Autodesk Inventor part; units mm, degrees
ref_plane "YZ Plane" through (0, 0, 0) normal (1, 0, 0) x (0, 1, 0)
ref_plane "XZ Plane" through (0, 0, 0) normal (0, 1, 0) x (-1, 0, 0)
ref_plane "XY Plane" through (0, 0, 0) normal (0, 0, 1) x (1, 0, 0)
sketch "Szkic1" plane through (0, 0, 0) normal (0, 0, 1) x (1, 0, 0)
  circle A0 centre (0, 0) radius 40
  circle A1 centre (0, 0) radius 53
  dimension "d0" = 80
  dimension "d1" = 13
extrude "Wyciągnięcie proste1" add sketch "Szkic1" along normal blind 5
sketch "Szkic2" plane through (0, 0, 5) normal (0, 0, 1) x (1, 0, 0)
  circle A0 centre (0, 0) radius 40
  circle A1 centre (0, 0) radius 43
  dimension "d4" = 3
extrude "Wyciągnięcie proste2" add sketch "Szkic2" along normal blind 41.5
sketch "Szkic3" plane through (0, 0, 5) normal (0, 0, 1) x (1, 0, 0)
  circle A0 centre (0, 0) radius 43
  line L0 (0, 43) -> (0, 53)
  circle A1 centre (0, 0) radius 53
  line L1 (43, 0) -> (53, 0)
  line L2 (0, -43) -> (0, -53)
  line L3 (-43, 0) -> (-53, 0)
  point P0 (0, 48)
  point P1 (-48, 0)
  point P2 (0, -48)
  point P3 (48, 0)
hole "Otwór1" at (0, 48, 5) at (-48, 0, 5) at (0, -48, 5) at (48, 0, 5) direction (0, 0, -1) diameter 3.242 end through all countersink diameter 8 countersink angle 90
sketch "Szkic8" plane through (0, 0, 0) normal (0, 0, -1) x (-1, 0, 0)
  circle A0 centre (0, 0) radius 10.75
  line L0 (0, 0) -> (17, 0)
  line L1 (17, 0) -> (14.59, 0)
  line L2 (14.59, 0) -> (14.59, 5)
  line L3 (14.59, 0) -> (14.59, -5)
  circle A1 centre (14.59, 5) radius 1.621
  circle A2 centre (14.59, -5) radius 1.621
  line L4 (14.59, 5) -> (-35.19, 5)
  line L5 (14.59, -5) -> (-35.19, -5)
  circle A3 centre (-35.19, 5) radius 1.621
  circle A4 centre (-35.19, -5) radius 1.621
  line L6 (-33.569, -5) -> (-31.569, -5)
  line L7 (-31.569, -5) -> (-31.569, 5)
  line L8 (-35.19, 6.621) -> (-35.19, 8.621)
  line L9 (-35.19, 8.621) -> (-31.569, 8.621)
  line L10 (-31.569, 8.621) -> (-31.569, 5)
  line L11 (-36.811, 5) -> (-38.811, 5)
  line L12 (-35.19, -6.621) -> (-35.19, -8.621)
  line L13 (-35.19, -8.621) -> (-31.569, -8.621)
  line L14 (-31.569, -8.621) -> (-31.569, -5)
  line L15 (-35.19, -8.621) -> (-38.811, -8.621)
  line L16 (-38.811, 5) -> (-38.811, 8.621)
  line L17 (-38.811, 8.621) -> (-35.19, 8.621)
  line L18 (12.969, -5) -> (10.969, -5)
  line L19 (14.59, -6.621) -> (14.59, -8.621)
  line L20 (10.969, -5) -> (10.969, -8.621)
  line L21 (10.969, -8.621) -> (14.59, -8.621)
  line L22 (14.59, 6.621) -> (14.59, 8.621)
  line L23 (14.59, 8.621) -> (10.969, 8.621)
  line L24 (10.969, 8.621) -> (10.969, -5)
  line L25 (16.211, -5) -> (18.211, -5)
  line L26 (14.59, -8.621) -> (18.211, -8.621)
  line L27 (18.211, -8.621) -> (18.211, 8.621)
  line L28 (18.211, 8.621) -> (14.59, 8.621)
  circle A5 centre (0, 0) radius 40
  line L29 (-38.811, -8.621) -> (-39.0599, -8.621)
  line L30 (-38.811, 8.621) -> (-39.0599, 8.621)
  line L31 (-31.569, 8.621) -> (-30.569, 8.621)
  line L32 (-30.569, 8.621) -> (-30.569, -8.621)
  line L33 (-30.569, -8.621) -> (-31.569, -8.621)
  dimension "d59" = 3.242
  dimension "d54" = 21.5
  dimension "d55" = 17
  dimension "d56" = 2.41
  dimension "d57" = 5
  dimension "d58" = 5
  dimension "d60" = 3.242
  dimension "d61" = 49.78
  dimension "d62" = 3.242
  dimension "d63" = 3.242
  dimension "d64" = 2
  dimension "d66" = 2
  dimension "d67" = 2
  dimension "d68" = 2
  dimension "d69" = 2
  dimension "d70" = 2
  dimension "d71" = 2
  dimension "d74" = 49.78
  dimension "d87" = 1
extrude "Wyciągnięcie proste6" add sketch "Szkic8" against normal blind 32 contours L24 L4 A1 L2 L0 | L0 L3 A2 L5 L24 | L24 L23 L22 A1 L4 | L5 A2 L19 L21 L20 | L2 A1 L22 L28 L27 L25 A2 L3 | L7 L5 A4 L12 L15 L29 A5 L30 L16 L11 A3 L4 | L4 A3 L8 L9 L10 | L14 L13 L12 A4 L5 | A2 L25 L27 L26 L19 | A3 L11 L16 L17 L8
sketch "Szkic9" plane through (0, 0, 0) normal (0, 0, -1) x (-1, 0, 0)
  line L0 (11.0032, 0) -> (10.969, -1.9997)
  line L1 (10.969, -8.621) -> (10.969, 8.621)
  line L2 (10.969, -1.9997) -> (10.969, 2.0003)
  line L3 (10.969, 2.0003) -> (-31.569, 2.0003)
  line L4 (-31.569, -8.621) -> (-31.569, 8.621)
  line L5 (10.969, -1.9997) -> (-31.569, -1.9997)
  circle A0 centre (14.59, -5) radius 1.621
  line L6 (14.59, -5) -> (14.59, -8.621)
  line L7 (18.211, -8.621) -> (10.969, -8.621)
  line L8 (14.59, -8.621) -> (12.59, -8.621)
  line L9 (12.59, -8.621) -> (16.59, -8.621)
  line L10 (16.59, -8.621) -> (16.59, -36.3974)
  arc A1 (-39.0599, -8.621) -> (-39.0599, 8.621) centre (0, 0) ccw
  line L11 (12.59, -8.621) -> (12.59, -37.967)
  line L12 (10.969, 8.621) -> (18.211, 8.621)
  line L13 (12.59, 8.621) -> (12.59, 45.8086)
  line L14 (12.59, 8.621) -> (49.7776, 8.621) construction
  line L15 (16.59, 8.621) -> (16.59, 43)
  point P0 (16.59, 36.3974)
  point P1 (12.59, 37.967)
  dimension "d75" = 2
  dimension "d76" = 4
  dimension "d77" = 2
  dimension "d78" = 4
  dimension "d79" = 90
extrude "Wyciągnięcie proste7" add sketch "Szkic9" against normal blind 3 contours L5 L4 L3 L1 | L7 L10 A1 L11 | L13 A1 L15 L12
equation "\"d62\" = d59"
equation "\"d63\" = d60"
equation "\"d74\" = d61"
properties part number "Podstawa1"
Read the model definition and answer for the solid it produces. Units are mm, in the model's axes. A direction names the side the tool comes from. Round coordinates to 2 decimals unless told otherwise and drop trailing zeros. Loops run counter-clockwise (first coordinate to the right, second up) from the corner with the lowest first, then second, coordinate; pieces in that order, holes last. Notation, with made-up numbers: (70.25, -33) -> (78.25, -33) arc R19 cw to (78.25, -23) -> close; hole circle Ø11 at (44, 17.25). An arc over 180 degrees is marked (long way). One line per item, written item: value.
1) A cutting plane is placed at C-C (x = 26). Determine the outline of the cut face in (y, z).
Answer list:
outline: (-46.18, 0) -> (-30.4, 0) -> (-30.4, 46.5) -> (-34.25, 46.5) -> (-34.25, 5) -> (-46.18, 5) -> close; (-2, 0) -> (2, 0) -> (2, 3) -> (-2, 3) -> close; (30.4, 0) -> (46.18, 0) -> (46.18, 5) -> (34.25, 5) -> (34.25, 46.5) -> (30.4, 46.5) -> close
2) For faces 1 (the face through (-15, 8.621, 16)), 2 (the face through (-12.59, -23, 1)), 3 (the face through (11, 1, 0)), determine the directions among +Z, -Z, +X, -X, +Y, -Y from which every point of the face is accessible in a straight line to the end or side of a thin tool.
Answer list:
face 1: +Z
face 2: +Z, -Z
face 3: -Z, +X, -X, +Y, -Y
3) A cutting plane is placed at A-A (z = 17). Determine the outline of the cut face in (x, y), and give its area (3 significant figures).
Answer list:
outline: circle Ø86 at (0, 0); (-18.21, -8.62) -> (-10.97, -8.62) -> (-10.97, 8.62) -> (-18.21, 8.62) -> close; hole circle Ø3.24 at (-14.59, -5); hole circle Ø3.24 at (-14.59, 5); hole (31.57, -8.62) -> (31.57, 8.62) -> (39.06, 8.62) arc R40 ccw (long way) to (39.06, -8.62) -> close; hole circle Ø3.24 at (35.19, -5); hole circle Ø3.24 at (35.19, 5)
area: 1,010 mm²
4) A cutting plane is placed at B-B (y = 48). Determine the outline of the cut face in (x, z), and give its area (3 significant figures).
Answer list:
outline: (-22.47, 0) -> (-1.62, 0) -> (-1.62, 2.62) -> (-4, 5) -> (-22.47, 5) -> close; (1.62, 0) -> (22.47, 0) -> (22.47, 5) -> (4, 5) -> (1.62, 2.62) -> close
area: 203 mm²
5) Consider L1, parallel to Y at x = 0, z = 24.5; L2, parallel to X at y = 2, z = 30; L3, parallel to X at y = 5.5, z = 6. Determine where each line is inside the solid, lowest interval first. Write a range as [from, to].
Answer list:
L1: y = [-43, -40], [40, 43]
L2: x = [-42.95, -39.95], [-18.21, -10.97], [31.57, 42.95]
L3: x = [-42.65, -39.62], [-18.21, -16.13], [-13.05, -10.97], [31.57, 33.65], [36.73, 42.65]
6) The mould has two halves that part along Y. Classify faces 4 (the face through (43, 4, 5)), 5 (the face through (36.476, -5.986, 15.776)), 6 (the face through (28, -45, 2)): pulls with the +Y half, pulls with the -Y half, needs draft (parallel to the pull), parting line crosses it, or undercut.
Answer list:
face 4: needs draft
face 5: undercut
face 6: parting line crosses it
7) Flat-ended cylindrical pins translate along their axes: P1, Ø3.5, axis at x = -14.5, z = 19, coming from the +Y side; P2, Ø3.5, axis at y = 27, z = 1, coming from the -X side; P3, Ø2, axis at y = -30.5, z = 41, coming from the +X side (3 decimals); P4, Ø3, axis at x = -48, y = 0, coming from the -Z side. Find the tip coordinate at first contact, or state that the pin passes through.
Answer list:
P1: stops at y = 41.07
P2: stops at x = -46.6
P3: stops at x = 31.285
P4: passes through
8) A cutting plane is placed at D-D (y = 10.5). Determine the outline of the cut face in (x, z).
Answer list:
outline: (-51.95, 0) -> (-38.6, 0) -> (-38.6, 46.5) -> (-41.7, 46.5) -> (-41.7, 5) -> (-51.95, 5) -> close; (-16.59, 0) -> (-12.59, 0) -> (-12.59, 3) -> (-16.59, 3) -> close; (38.6, 0) -> (51.95, 0) -> (51.95, 5) -> (41.7, 5) -> (41.7, 46.5) -> (38.6, 46.5) -> close
